Design review of the part built by this model. Coordinates are the model's own, in mm. Face numbers are marked on the shaded views. A direction names the side the tool comes from. Coordinates: 2 decimals unless noted, no trailing zeros. Answer in a Markdown table with one row per item. Add a question column.
Item 1: Take a section at B-B, the plane y = 216. Give the number of separate pieces and of enclosed holes in the cut face, and give its area (3 significant figures).
Item 2: To check wall thickness, follow line 1 (Y direction, x = -16, z = -25.5); line 2 (X direction, y = 207.5, z = -57.15) (1 decimal); line 3 (Y direction, x = 38, z = -48.5). State the ranges of each line that lie inside material, in increasing order.
Item 3: For the marked faces 1, 2, 3, 4 and 5, list the 3-axis set-ups (+Z, -Z, +X, -X, +Y, -Y) from which the entire face can be reached by the end or side of a thin tool; tool diameter is ignored.
Item 4: Draft analysis for pull direction Z (two halves, no side actions). For the marked faces 6, 7 and 8, state which applies: released by +Z, released by -Z, zero draft, split by the parting line, or undercut.
Item 5: Clearance check with flat-ended pins moving along their axes: P1, Ø4, axis at x = 17, z = -20, coming from the +Y side; P2, Ø5.5, axis at x = -39.5, z = -52, coming from the +Y side; P3, Ø5, axis at y = 159, z = -42.5, coming from the +X side. State where each tip first meets the part, or that it passes through.
from build123d import *

# Parameters (mm, degrees)
BOSS_EXTRUDE1_DEPTH  = 139.7
SHELL1_T             = -1.5875
BOSS_EXTRUDE2_DEPTH  = 1.5875
SKETCH3_R            = 31.75
BOSS_EXTRUDE3_DEPTH  = 6.35
SKETCH4_R            = 44.45
BOSS_EXTRUDE4_DEPTH  = 3.175
BOSS_EXTRUDE5_DEPTH  = 6.35
SKETCH6_R            = 36.5125
BOSS_EXTRUDE6_DEPTH  = 25.4
SKETCH8_R            = 38.1
BOSS_EXTRUDE7_DEPTH  = 19.05
SKETCH9_R            = 39.6875
BOSS_EXTRUDE8_DEPTH  = 1.5875
SKETCH10_R           = 38.1
SKETCH10_R_2         = 36.5125
BOSS_EXTRUDE9_DEPTH  = 6.35
SKETCH12_R           = 34.925
SKETCH12_R_2         = 33.3375
BOSS_EXTRUDE10_DEPTH = 19.05
SKETCH15_R           = 14.2875
CUT_EXTRUDE1_DEPTH   = 19.05


with BuildPart() as part:
    # Sketch1 → Boss-Extrude1 (new body)
    with BuildSketch(Plane(origin=(0, 0, 0), x_dir=(1, 0, 0), z_dir=(0, 1, 0))):
        with BuildLine():
            Line((-41.275, 0), (41.275, 0))
            Line((41.275, 0), (41.275, 57.15))
            ThreePointArc((41.275, 57.15), (0, 98.425), (-41.275, 57.15))
            Line((-41.275, 57.15), (-41.275, 0))
        make_face()
    extrude(amount=BOSS_EXTRUDE1_DEPTH)

    # Shell1
    shell1_openings = [part.faces().sort_by_distance(p)[0] for p in [
        (0, 139.7, -45.257423889),
    ]]
    offset(amount=SHELL1_T, openings=shell1_openings, kind=Kind.INTERSECTION)

    # Sketch2 → Boss-Extrude2 (add)
    with BuildSketch(Plane(origin=(0, 139.7, 0), x_dir=(1, 0, 0), z_dir=(0, 1, 0))):
        with BuildLine():
            Line((41.275, 0), (41.275, 57.15))
            ThreePointArc((41.275, 57.15), (0, 98.425), (-41.275, 57.15))
            Line((-41.275, 57.15), (-41.275, 0))
            Line((-41.275, 0), (41.275, 0))
        make_face()
    extrude(amount=BOSS_EXTRUDE2_DEPTH)

    # Sketch3 → Boss-Extrude3 (add)
    with BuildSketch(Plane(origin=(0, 141.2875, 0), x_dir=(1, 0, 0), z_dir=(0, 1, 0))):
        with Locations(Location((0, 57.15, 0), (0, 0, 270))):
            Circle(SKETCH3_R)
    extrude(amount=BOSS_EXTRUDE3_DEPTH)

    # Sketch4 → Boss-Extrude4 (add)
    with BuildSketch(Plane(origin=(0, 147.6375, 0), x_dir=(1, 0, 0), z_dir=(0, 1, 0))):
        with Locations(Location((0, 57.15, 0), (0, 0, 270))):
            Circle(SKETCH4_R)
    extrude(amount=BOSS_EXTRUDE4_DEPTH)

    # Sketch5 → Boss-Extrude5 (add)
    with BuildSketch(Plane(origin=(0, 150.8125, 0), x_dir=(1, 0, 0), z_dir=(0, 1, 0))):
        with BuildLine():
            ThreePointArc((-3.805939848, 98.249153846), (-20.6375, 92.895198541), (-33.689941381, 80.995617517))
            ThreePointArc((-33.689941381, 80.995617517), (-39.04475533, 79.6925), (-37.495881229, 74.403536329))
            ThreePointArc((-37.495881229, 74.403536329), (-41.275, 57.15), (-37.495881229, 39.896463671))
            ThreePointArc((-37.495881229, 39.896463671), (-39.04475533, 34.6075), (-33.689941381, 33.304382483))
            ThreePointArc((-33.689941381, 33.304382483), (-20.6375, 21.404801459), (-3.805939848, 16.050846154))
            ThreePointArc((-3.805939848, 16.050846154), (0, 12.065), (3.805939848, 16.050846154))
            ThreePointArc((3.805939848, 16.050846154), (20.6375, 21.404801459), (33.689941381, 33.304382483))
            ThreePointArc((33.689941381, 33.304382483), (39.04475533, 34.6075), (37.495881229, 39.896463671))
            ThreePointArc((37.495881229, 39.896463671), (41.275, 57.15), (37.495881229, 74.403536329))
            ThreePointArc((37.495881229, 74.403536329), (39.04475533, 79.6925), (33.689941381, 80.995617517))
            ThreePointArc((33.689941381, 80.995617517), (20.6375, 92.895198541), (3.805939848, 98.249153846))
            ThreePointArc((3.805939848, 98.249153846), (0, 102.235), (-3.805939848, 98.249153846))
        make_face()
    extrude(amount=BOSS_EXTRUDE5_DEPTH)

    # Sketch6 → Boss-Extrude6 (add)
    with BuildSketch(Plane(origin=(0, 157.1625, 0), x_dir=(1, 0, 0), z_dir=(0, 1, 0))):
        with Locations(Location((0, 57.15, 0), (0, 0, 270))):
            Circle(SKETCH6_R)
    extrude(amount=BOSS_EXTRUDE6_DEPTH)

    # Sketch8 → Boss-Extrude7 (add)
    with BuildSketch(Plane(origin=(0, 182.5625, 0), x_dir=(1, 0, 0), z_dir=(0, 1, 0))):
        with Locations(Location((0, 57.15, 0), (0, 0, 90))):
            Circle(SKETCH8_R)
    extrude(amount=BOSS_EXTRUDE7_DEPTH)

    # Sketch9 → Boss-Extrude8 (add)
    with BuildSketch(Plane(origin=(0, 201.6125, 0), x_dir=(1, 0, 0), z_dir=(0, 1, 0))):
        with Locations(Location((0, 57.15, 0), (0, 0, 270))):
            Circle(SKETCH9_R)
    extrude(amount=BOSS_EXTRUDE8_DEPTH)

    # Sketch10 → Boss-Extrude9 (add)
    with BuildSketch(Plane(origin=(0, 203.2, 0), x_dir=(1, 0, 0), z_dir=(0, 1, 0))):
        with Locations(Location((0, 57.15, 0), (0, 0, 90))):
            Circle(SKETCH10_R)
        with Locations(Location((0, 57.15, 0), (0, 0, 270))):
            Circle(SKETCH10_R_2, mode=Mode.SUBTRACT)
    extrude(amount=BOSS_EXTRUDE9_DEPTH)

    # Sketch12 → Boss-Extrude10 (add)
    with BuildSketch(Plane(origin=(0, 203.2, 0), x_dir=(1, 0, 0), z_dir=(0, 1, 0))):
        with Locations(Location((0, 57.15, 0), (0, 0, 90))):
            Circle(SKETCH12_R)
        with Locations(Location((0, 57.15, 0), (0, 0, 90))):
            Circle(SKETCH12_R_2, mode=Mode.SUBTRACT)
    extrude(amount=BOSS_EXTRUDE10_DEPTH)

    # Sketch14 → Revolve1 (revolve)
    with BuildSketch(Plane(origin=(0, 0, 0), x_dir=(0, 0, -1), z_dir=(1, 0, 0)), mode=Mode.PRIVATE) as revolve1_sk:
        Polygon((57.15, 238.125), (76.2, 238.125), (76.2, 225.425), (82.55, 223.8375), (82.55, 203.2), (57.15, 203.2), align=None)
    revolve(revolve1_sk.sketch.rotate(Axis((0, 235.492882867, -57.15), (0, -1, 0)), 180), axis=Axis((0, 235.492882867, -57.15), (0, -1, 0)))

    # Sketch15 → Cut-Extrude1 (cut)
    with BuildSketch(Plane(origin=(0, 238.125, 0), x_dir=(1, 0, 0), z_dir=(0, 1, 0))):
        with Locations(Location((0, 57.15, 0), (0, 0, 270))):
            Circle(SKETCH15_R)
    extrude(amount=-CUT_EXTRUDE1_DEPTH, mode=Mode.SUBTRACT)


solid = part.part
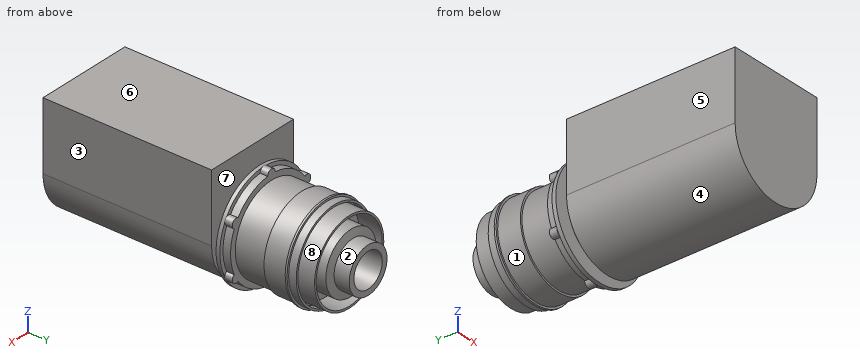
Answers:
| question | item | result |
|---|---|---|
| 1 | separate pieces | 2 |
| 1 | enclosed holes | 1 |
| 1 | area | 2,370 mm^2 |
| 2 | line 1 | y = 0 to 1.59, 139.7 to 141.29, 147.64 to 203.2 |
| 2 | line 2 | x = -38.1 to -36.5, -34.9 to -33.3, -25.4 to 25.4, 33.3 to 34.9, 36.5 to 38.1 |
| 2 | line 3 | y = 0 to 1.59, 139.7 to 141.29, 147.64 to 157.16, 201.61 to 203.2 |
| 3 | face 1 | none |
| 3 | face 2 | +Y |
| 3 | face 3 | +Z, -Z, +X, -Y |
| 3 | face 4 | -Z, -Y |
| 3 | face 5 | +Z, -Z, -X, -Y |
| 4 | face 6 | released by +Z |
| 4 | face 7 | zero draft |
| 4 | face 8 | undercut |
| 5 | P1 | stops at y = 203.2 |
| 5 | P2 | stops at y = 209.55 |
| 5 | P3 | stops at x = 39.19 |
